from build123d import *

# Parameters (mm, degrees)
EXTRUDE_1_DEPTH = 5
FILLET_1_R      = 1.5


with BuildPart() as part:
    # 草图1 → 凸台-拉伸1 (new body)
    with BuildSketch(Plane(origin=(0, 0, 0), x_dir=(1, 0, 0), z_dir=(0, 1, 0))):
        Polygon((6.25, -9.219059406), (-6.25, -9.219059406), (-6.25, -6.219059406), (-17.5, -6.219059406), (-17.5, -9.219059406), (-30, -9.219059406), (-30, -6.219059406), (-35, -6.219059406), (-35, 8.780940594), (-26.25, 20.280940594), (-20, 20.280940594), (-20, 23.280940594), (-7.5, 23.280940594), (-7.5, 20.280940594), (7.5, 20.280940594), (7.5, 23.280940594), (20, 23.280940594), (20, 20.280940594), (26.25, 20.280940594), (35, 8.780940594), (35, -6.219059406), (30, -6.219059406), (30, -9.219059406), (17.5, -9.219059406), (17.5, -6.219059406), (6.25, -6.219059406), align=None)
        Polygon((-29, 6.757846183), (-24.718664622, 12.384744108), (-6.718567757, -0.219059406), (-29, -0.219059406), align=None, mode=Mode.SUBTRACT)
        Polygon((-18.709479877, 14.280940594), (-2.5, 2.930940594), (-2.5, 14.280940594), align=None, mode=Mode.SUBTRACT)
        Polygon((2.5, 14.280940594), (18.709479877, 14.280940594), (2.5, 2.930940594), align=None, mode=Mode.SUBTRACT)
        Polygon((6.718567757, -0.219059406), (24.718664622, 12.384744108), (29, 6.757846183), (29, -0.219059406), align=None, mode=Mode.SUBTRACT)
    extrude(amount=EXTRUDE_1_DEPTH)

    # 圆角1
    fillet_1_edges = [part.edges().sort_by_distance(p)[0] for p in [
        (29, 2.5, 0.219059406),
        (29, 2.5, -6.757846183),
        (24.718664622, 2.5, -12.384744108),
        (-2.5, 2.5, -14.280940594),
        (-18.709479877, 2.5, -14.280940594),
        (-2.5, 2.5, -2.930940594),
        (-6.718567757, 2.5, 0.219059406),
        (-24.718664622, 2.5, -12.384744108),
        (-29, 2.5, -6.757846183),
        (-29, 2.5, 0.219059406),
        (2.5, 2.5, -14.280940594),
        (2.5, 2.5, -2.930940594),
        (18.709479877, 2.5, -14.280940594),
        (6.718567757, 2.5, 0.219059406),
    ]]
    fillet(fillet_1_edges, radius=FILLET_1_R)


solid = part.part
Build history of the part. All positions in model axes, mm. A direction names the side the tool comes from. Coordinates: 2 decimals unless noted, no trailing zeros. Order: outer loops, then holes, each group sorted by start corner. A loop starts at its lowest first (then second) coordinate and runs counter-clockwise, first axis right, second up. Notation, with made-up numbers: (42, 0) -> (62, 0) arc R28 ccw to (62, 27) -> close; hole circle Ø8 at (-15.5, 60). An arc over 180 degrees is marked (long way). One line per item, written item: value.
(1) Slice it at C-C, the plane y = 1.75. Count the separate pieces of the cut face and the enclosed holes in it, plus the area to 3 significant figures.
Checked values:
separate pieces: 1
enclosed holes: 4
area: 1,470 mm2
(2) Slice it at B-B, the plane z = -8. List the corners of the cut face in (x, y), plus the area to 3 significant figures.
Checked values:
outline: (-35, 0) -> (-28.05, 0) -> (-28.05, 5) -> (-35, 5) -> close; (-18.46, 0) -> (-9.74, 0) -> (-9.74, 5) -> (-18.46, 5) -> close; (-2.5, 0) -> (2.5, 0) -> (2.5, 5) -> (-2.5, 5) -> close; (9.74, 0) -> (18.46, 0) -> (18.46, 5) -> (9.74, 5) -> close; (28.05, 0) -> (35, 0) -> (35, 5) -> (28.05, 5) -> close
area: 182 mm2
(3) Mould opens along X. For faces 1 (the flat face through (-24, 2, 9.219)), 2 (the flat face through (9, 2, -14.281)), 3 (the flat face through (30.564, 2.465, -14.611)) say: pulls with the +X half, pulls with the -X half, needs draft (parallel to the pull), parting line crosses it, or undercut.
Checked values:
face 1: needs draft
face 2: undercut
face 3: pulls with the +X half
(4) Probe line 1 (X direction, y = 2.5, z = -7); line 2 (X direction, y = 2.85, z = -11.5); line 3 (X direction, y = 3.9, z = -13.5). List the from-to ranges inside material, lowest first. Write a range as [from, to].
Checked values:
line 1: [-35, -28.8], [-17.03, -8.31], [-2.5, 2.5], [8.31, 17.03], [28.8, 35]
line 2: [-32.93, -25.34], [-23.46, -14.74], [-2.5, 2.5], [14.74, 23.46], [25.34, 32.93]
line 3: [-31.41, -15.27], [-2.68, 2.68], [15.27, 31.41]
(5) Tool access for faces 4 (the flat face through (27.12, 2.46, -9.23)), 5 (the flat face through (-7.5, 2, -22)), 6 (the flat face through (-17.5, 2, 8)): list every direction of +Z, -Z, +X, -X, +Y, -Y with a clear straight run to the whole face (end or side of a thin tool).
Checked values:
face 4: +Y, -Y
face 5: -Z, +Y, -Y
face 6: +Z, +Y, -Y
(6) Drop flat-ended pins along their axis: pin 1 Ø0.9 at (y, z) = (1.5, -21.5) entering from -X; pin 2 Ø1.5 at (x, y) = (31.5, 3) entering from +Z; pin 3 Ø0.9 at (y, z) = (2, 7) entering from -X. Give the stop position or say it passes through.
Checked values:
pin 1: x = -20
pin 2: z = 6.22
pin 3: x = -30
(7) Slice it at A-A, the plane x = -16.5. List the corners of the cut face in (y, z).
Checked values:
outline: (0, -23.28) -> (5, -23.28) -> (5, -6.63) -> (0, -6.63) -> close; (0, 0.22) -> (5, 0.22) -> (5, 6.22) -> (0, 6.22) -> close
